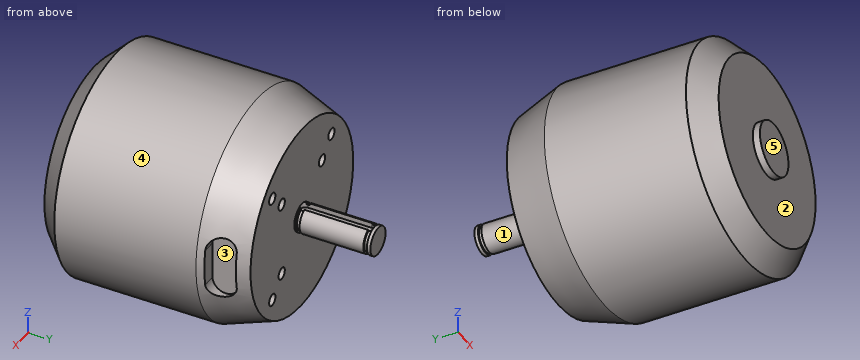
from build123d import *

# Parameters (mm, degrees)
M4X0_7_1_D          = 3.3
M4X0_7_1_DEPTH      = 11.5
M4X0_7_1_TIP        = 0.991420021
CUT_EXTRUDE1_DEPTH  = 1.8
CHAMFER_1_SIZE      = 4.5
CHAMFER_1_SIZE2     = 13
CHAMFER_2_SIZE      = 6
SKETCH_6_R          = 7.5
EXTRUDE_1_DEPTH     = 2
SKETCH_7_W          = 0.5
SKETCH_7_H          = 1
CUT_EXTRUDE_START   = 31.5
CUT_EXTRUDE_1_DEPTH = 5


with BuildPart() as part:
    # 스케치1 → 회전1 (revolve)
    with BuildSketch(Plane.XY, mode=Mode.PRIVATE) as revolve_1_sk:
        Polygon((0, 80.5), (4, 80.5), (4, 59), (31.5, 59), (31.5, 0), (0, 0), align=None)
    revolve(revolve_1_sk.sketch.rotate(Axis((0, 0, 0), (0, 1, 0)), 90), axis=Axis((0, 0, 0), (0, 1, 0)))

    # M4x0.7 나사 구멍1
    with Locations(Plane(origin=(0, 59, 0), x_dir=(1, 0, 0), z_dir=(0, 1, 0))):
        with Locations((10.606601718, 10.606601718), (15.556349186, 15.556349186), (10.606601718, -10.606601718), (15.556349186, -15.556349186), (-10.606601718, -10.606601718), (-15.556349186, -15.556349186), (-10.606601718, 10.606601718), (-15.556349186, 15.556349186)):
            Hole(M4X0_7_1_D / 2, depth=M4X0_7_1_DEPTH)
            with Locations((0, 0, -(M4X0_7_1_DEPTH + M4X0_7_1_TIP / 2))):  # 118° drill point
                Cone(0, M4X0_7_1_D / 2, M4X0_7_1_TIP, mode=Mode.SUBTRACT)

    # Sketch3 → Cut-Extrude1 (cut)
    with BuildSketch(Plane(origin=(2.845698698, 80.5, 4), x_dir=(0, 1, 0), z_dir=(0, 0, -1))):
        with BuildLine():
            Line((-2.5, -1.345698698), (-20.5, -1.345698698))
            ThreePointArc((-20.5, -1.345698698), (-22, -2.845698698), (-20.5, -4.345698698))
            Line((-20.5, -4.345698698), (-2.5, -4.345698698))
            ThreePointArc((-2.5, -4.345698698), (-1, -2.845698698), (-2.5, -1.345698698))
        make_face()
    extrude(amount=CUT_EXTRUDE1_DEPTH, mode=Mode.SUBTRACT)

    # 모따기1
    chamfer_1_edges = [part.edges().sort_by_distance(p)[0] for p in [
        (0, 59, 31.5),
    ]]
    chamfer_1_side = [part.faces().sort_by_distance(p)[0] for p in [
        (0, 59, 30.609045456),
    ]]
    chamfer(chamfer_1_edges, length=CHAMFER_1_SIZE, length2=CHAMFER_1_SIZE2, reference=chamfer_1_side[0])

    # 모따기2
    chamfer_2_edges = [part.edges().sort_by_distance(p)[0] for p in [
        (0, 0, 31.5),
    ]]
    chamfer(chamfer_2_edges, length=CHAMFER_2_SIZE)

    # 스케치6 → 보스-돌출1 (add)
    with BuildSketch(Plane.XZ):
        with Locations(Location((0, 0, 0), (0, 0, 270))):
            Circle(SKETCH_6_R)
    extrude(amount=EXTRUDE_1_DEPTH)

    # 스케치7 → 컷-회전1 (revolve, cut)
    with BuildSketch(Plane(origin=(0, 0, 0), x_dir=(0, 0, -1), z_dir=(1, 0, 0))):
        with Locations((3.75, 79)):
            Rectangle(SKETCH_7_W, SKETCH_7_H)
        with Locations((3.75, 60)):
            Rectangle(SKETCH_7_W, SKETCH_7_H)
    revolve(axis=Axis((0, 0, 0), (0, 1, 0)), mode=Mode.SUBTRACT)

    # 스케치9 → 컷-돌출1 (cut)
    with BuildSketch(Plane(origin=(0, 0, 0), x_dir=(0, 0, -1), z_dir=(1, 0, 0)).offset(CUT_EXTRUDE_START)):
        with BuildLine():
            Line((5.25, 48), (-5.25, 48))
            ThreePointArc((-5.25, 48), (-9, 51.75), (-5.25, 55.5))
            Line((-5.25, 55.5), (5.25, 55.5))
            ThreePointArc((5.25, 55.5), (9, 51.75), (5.25, 48))
        make_face()
    extrude(amount=-CUT_EXTRUDE_1_DEPTH, mode=Mode.SUBTRACT)


solid = part.part
Read the model definition and answer for the solid it produces. Units are mm, in the model's axes. Face numbers are marked on the shaded views. A direction names the side the tool comes from. Give positions to 0.01 mm unless a question says otherwise; leave off trailing zeros. Write each loop counter-clockwise with the first axis right and the second up, starting at its lowest first coordinate (ties: lowest second). Pieces come first, ordered by that corner, then holes. Notation, with made-up numbers: (58.25, 77) - (91.25, 77) arc R11 ccw to (91.25, 93) - close; hole circle Ø5 at (82.25, -16). An arc over 180 degrees is marked (long way). Use CSV: the item, a comma, the result in double quotes. Start each with the question number.
Item 1: Consider line 1 (Y direction, x = -5, z = -19); line 2 (X direction, y = 15.5, z = 0.5); line 3 (Z direction, x = 21, y = 4.5). Determine where each line is inside the solid, lowest interval first.
Item 2: The part is cut by section B-B, the plane y = 72.5. Give the vertices of the cut face in (x, z).
Item 3: The mould has two halves that part along Y. Classify the marked faces 3, 4 and 5: pulls with the +Y half, pulls with the -Y half, needs draft (parallel to the pull), parting line crosses it, or undercut.
Item 4: Flat-ended cylindrical pins translate along their axes: P1, Ø4, axis at y = 9, z = 21.5, coming from the -X side; P2, Ø4.5, axis at x = 15.56, z = -15.56, coming from the -Y side; P3, Ø2.5, axis at x = -10.61, z = -10.61, coming from the +Y side. Find the tip coordinate at first contact, or state that the pin passes through.
Item 5: The part is cut by section A-A, the plane y = 23. Give the vertices of the cut face in (x, z).
Item 6: For the marked faces 1 and 2, determine the directions among +Z, -Z, +X, -X, +Y, -Y from which every point of the face is accessible in a straight line to the end or side of a thin tool.
Taken from the geometry:
1,line 1,"0 to 59"
1,line 2,"-31.5 to 31.5"
1,line 3,"-21.42 to 21.42"
2,outline,"(-1.5, 2.2) - (-1.5, 3.71) arc R4 ccw (long way) to (1.5, 3.71) - (1.5, 2.2) - close"
3,face 3,"undercut"
3,face 4,"needs draft"
3,face 5,"pulls with the -Y half"
4,P1,"x = -24.74"
4,P2,"y = 0"
4,P3,"y = 47.26"
5,outline,"circle Ø63 at (0, 0)"
6,face 1,"+Y"
6,face 2,"-Y"
